Design review of the part built by this model. Coordinates are the model's own, in mm. Give positions to 0.01 mm unless a question says otherwise; leave off trailing zeros. Answer as CSV lines item,"result".
```python
from build123d import *

# Parameters (mm, degrees)
SKETCH_1_R      = 1.5
EXTRUDE_1_DEPTH = 6


with BuildPart() as part:
    # 草图1 → 凸台-拉伸1 (new body)
    with BuildSketch(Plane(origin=(0, 0, 0), x_dir=(1, 0, 0), z_dir=(0, 1, 0))):
        with BuildLine():
            Line((-112.725, 113.5), (-7.662552173, 113.5))
            ThreePointArc((-7.662552173, 113.5), (-0.28, 106.117447827), (7.102552173, 113.5))
            Line((7.102552173, 113.5), (7.5, 113.5))
            Line((7.5, 113.5), (117.725, 113.5))
            Line((117.725, 113.5), (117.725, -113.5))
            Line((117.725, -113.5), (-112.725, -113.5))
            Line((-112.725, -113.5), (-112.725, 113.5))
        make_face()
        with Locations(Location((-92.725, 93.5, 0), (0, 0, 270))):
            Circle(SKETCH_1_R, mode=Mode.SUBTRACT)
        with Locations(Location((97.725, 93.5, 0), (0, 0, 270))):
            Circle(SKETCH_1_R, mode=Mode.SUBTRACT)
        with Locations(Location((2.5, 93.5, 0), (0, 0, 270))):
            Circle(SKETCH_1_R, mode=Mode.SUBTRACT)
        with Locations(Location((-92.725, -83.5, 0), (0, 0, 270))):
            Circle(SKETCH_1_R, mode=Mode.SUBTRACT)
        with Locations(Location((2.5, -83.5, 0), (0, 0, 270))):
            Circle(SKETCH_1_R, mode=Mode.SUBTRACT)
        with Locations(Location((92.725, -83.5, 0), (0, 0, 270))):
            Circle(SKETCH_1_R, mode=Mode.SUBTRACT)
    extrude(amount=EXTRUDE_1_DEPTH)


solid = part.part
```
1. For P1, Ø3.5, axis at x = 2.5, z = -93.5, coming from the +Y side; P2, Ø2.5, axis at x = -92.725, z = 83.5, coming from the -Y side, all flat-tipped, find the tip position at first contact; note any pin that passes through.
Answer block:
P1,"y = 6"
P2,"through"
2. The part is to be moulded in two halves that separate along X. For faces 1 (the cylindrical face through (-0.44, 2.96, -106.12)), 2 (the flat face through (-112.725, 3, 2)), 3 (the flat face through (-61, 3, -113.5)), say which applies: pulls with the +X half, pulls with the -X half, needs draft (parallel to the pull), parting line crosses it, or undercut.
Answer block:
face 1,"undercut"
face 2,"pulls with the -X half"
face 3,"needs draft"
3. To check wall thickness, follow L1, parallel to Z at x = -93, y = 2.85; L2, parallel to X at y = 3.8, z = 83.5 (3 decimals); L3, parallel to X at y = 3.25, z = -93.5 (3 decimals). State the ranges of each line that lie inside material, in increasing order. Write a range as [from, to].
Answer block:
L1,"[-113.5, -94.97], [-92.03, 82.03], [84.97, 113.5]"
L2,"[-112.725, -94.225], [-91.225, 1], [4, 91.225], [94.225, 117.725]"
L3,"[-112.725, -94.225], [-91.225, 1], [4, 96.225], [99.225, 117.725]"
